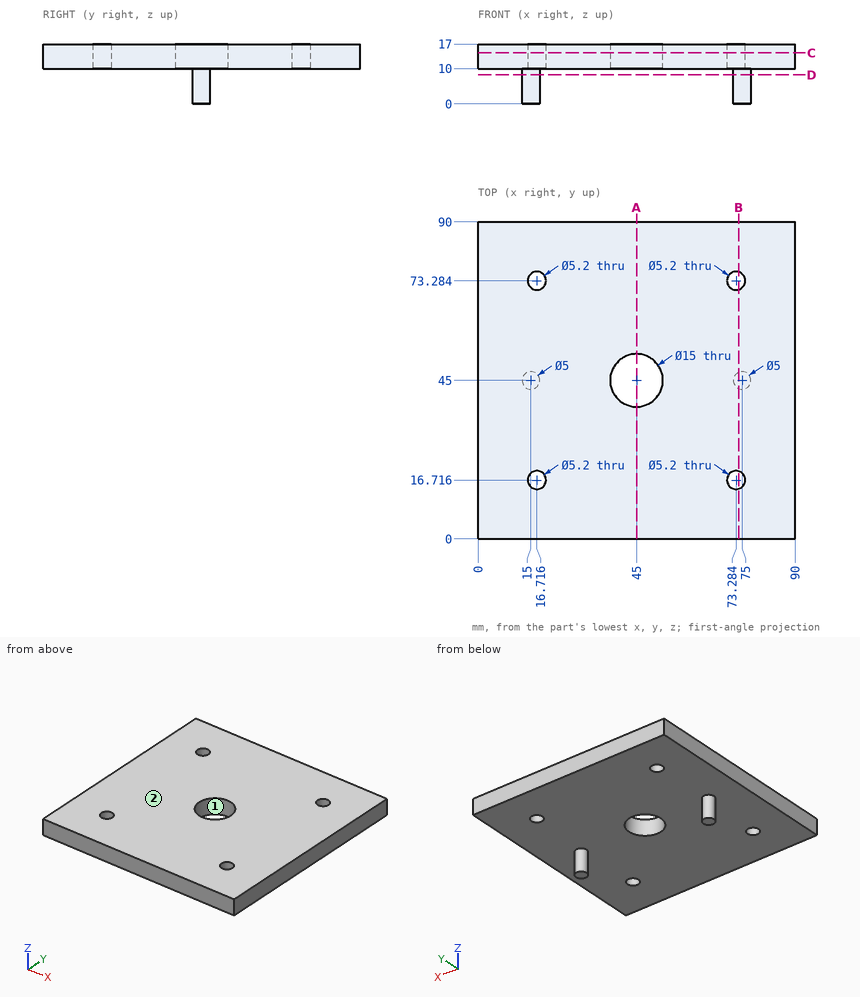
Input: dimensioned drawing with shaded views. Units: mm. Origin: part minimum x, y, z. Coordinates: 2 decimals unless noted, no trailing zeros. Write each loop counter-clockwise with the first axis right and the second up, starting at its lowest first coordinate (ties: lowest second). Pieces come first, ordered by that corner, then holes. Notation, with made-up numbers: M 87,42.5 L 102,42.5 A32 ccw 102,70.5 Z; hole C 61,-26.5 d11. An arc over 180 degrees is marked long. Answer as CSV lines item,"result". Start each with the question number.
Q1. Cut plane A-A on x = 45. Return the cut outline in (y, z).
Q2. Mould query, pull axis Y, two halves, no side actions, for the marked faces 1 and 2. Classes: released by +Y, released by -Y, zero draft, split by the parting line, or undercut.
Q3. Cut plane C-C on z = 14.5. Return the cut outline in (x, y).
Q4. Line query: line 1 (Y direction, x = 72, z = 15.5) (1 decimal); line 2 (Z direction, x = 76.5, y = 20.5); line 3 (Y direction, x = 48.5, z = 14.5). Output: solid intervals per line, ascending. Write a range as from..to.
Q5. Pin query (flat end, axial travel): P1, Ø7, axis at x = 73.28, y = 16.72, coming from the -Z side. Return the tip coordinate at first contact, or that it passes through.
Q6. Cut plane D-D on z = 8.25. Return the cut outline in (x, y).
Q7. Cut plane B-B on x = 74. Return the cut outline in (y, z) (1 decimal), then the cut area to 3 significant figures.
Findings below:
1,outline,"M 0,10 L 37.5,10 L 37.5,17 L 0,17 Z; M 52.5,10 L 90,10 L 90,17 L 52.5,17 Z"
2,face 1,"undercut"
2,face 2,"zero draft"
3,outline,"M 0,0 L 90,0 L 90,90 L 0,90 Z; hole C 16.72,16.72 d5.2; hole C 16.72,73.28 d5.2; hole C 45,45 d15; hole C 73.28,16.72 d5.2; hole C 73.28,73.28 d5.2"
4,line 1,"y = 0..14.5, 19..71, 75.5..90"
4,line 2,"z = 10..17"
4,line 3,"y = 0..38.37, 51.63..90"
5,P1,"stops at z = 10"
6,outline,"C 15,45 d5; C 75,45 d5"
7,outline,"M 0,10 L 14.2,10 L 14.2,17 L 0,17 Z; M 19.2,10 L 42.7,10 L 42.7,0 L 47.3,0 L 47.3,10 L 70.8,10 L 70.8,17 L 19.2,17 Z; M 75.8,10 L 90,10 L 90,17 L 75.8,17 Z"
7,area,"606 mm2"
